Source: CAD feature listing. Evaluate the final solid. Frame: model axes, mm. A direction names the side the tool comes from. Coordinates: 2 decimals unless noted, no trailing zeros. Write each loop counter-clockwise with the first axis right and the second up, starting at its lowest first coordinate (ties: lowest second). Pieces come first, ordered by that corner, then holes. Notation, with made-up numbers: M 68,44.25 L 102,44.25 A24 cw 102,56.25 Z; hole C -28,79 d6. An arc over 180 degrees is marked long. Write item = value, one per line. Start each with the question number.
1. Section query A-A (z = 9.75). Output: boundary loops of the cut face in (x, y).
2. Pin query (flat end, axial travel): pin 1 Ø17.5 at (y, z) = (-6.5, 8.5) entering from +X; pin 2 Ø11 at (x, z) = (3.5, -5) entering from -Y; pin 3 Ø13 at (x, z) = (14, -4) entering from +Y; pin 4 Ø6 at (y, z) = (-43, 1) entering from -X. Return the tip coordinate at first contact, or that it passes through.
3. Section query D-D (z = -7.75). Output: boundary loops of the cut face in (x, y).
4. Pull-direction query (X, two-part tool) for faces 1 (the face through (59, -16.4, 1)), 2 (the face through (82.6, 20.5, 1.6)), 3 (the face through (48.612, 22.153, 1.158)); classes: pulls with the +X half, pulls with the -X half, needs draft (parallel to the pull), parting line crosses it, or undercut.
5. Line query: line 1 along X through (y, z) = (-21.5, 8.5); line 2 along Y through (x, z) = (35, -8); line 3 along Z through (x, y) = (57, 6). Output: solid intervals per line, ascending.
6. Section query B-B (x = 44). Output: boundary loops of the cut face in (y, z), then the cut area to 3 significant figures.
7. Section query C-C (y = -82.5). Output: boundary loops of the cut face in (x, z), then the cut area to 3 significant figures.
8. Access query for faces 4 (the face through (81.4, -20.5, 1.6)), 5 (the face through (88, 24, 10)), 6 (the face through (-59, -16.4, 1)). Directions: +Z, -Z, +X, -X, +Y, -Y. A direction counts if a zero-diameter tool reaches every point of the face in a straight line with its end or side. Return the directions, or none.
```python
from build123d import *

# Parameters (mm, degrees)
F0_W      = 56
F0_H      = 16
F1_DEPTH  = 27.5
F2_DEPTH  = 15
F4_DEPTH  = 30.001
F6_DEPTH  = 18
F9_D      = 2.5
F9_DEPTH  = 12
F9_TIP    = 0.7510757738
F11_DEPTH = 2


with BuildPart() as f1:
    # F0 (on Front) → F1 (new body, symmetric)
    with BuildSketch(Plane.XZ):
        Polygon((-30, 20), (-90, 20), (-90, 0), (-55, 0), (-30, 0), align=None)
        with Locations((-60, 10)):
            Rectangle(F0_W, F0_H, mode=Mode.SUBTRACT)
    extrude(amount=F1_DEPTH, both=True)


with BuildPart() as f1b:
    # F0 (on Front) → F1, piece 2 (new body, symmetric)
    with BuildSketch(Plane.XZ):
        Polygon((30, 20), (30, 0), (55, 0), (90, 0), (90, 20), align=None)
        with Locations((60, 10)):
            Rectangle(F0_W, F0_H, mode=Mode.SUBTRACT)
    extrude(amount=F1_DEPTH, both=True)


with BuildPart() as f2:
    # F0 (on Front) → F2 (new body, symmetric)
    with BuildSketch(Plane.XZ):
        Polygon((30, 0), (-30, 0), (-55, 0), (-55, -1), (-46, -10), (46, -10), (55, -1), (55, 0), align=None)
    extrude(amount=F2_DEPTH, both=True)

    # F10 (on face) → F11 (join)
    with BuildSketch(Plane.XY):
        Polygon((28.5, 15), (-28.5, 15), (-28.5, -27), (-19.5, -78), (-19.5, -115), (19.5, -115), (19.5, -78), (28.5, -27), align=None)
    extrude(amount=F11_DEPTH)


with BuildPart() as f4_tool:
    # F3 (on face) → F4 (new body, through all)
    with BuildSketch(Plane.XY.offset(20)):
        Polygon((-30, 27.5), (-70, 27.5), (-30, 17.5), align=None)
        Polygon((-70, -27.5), (-30, -27.5), (-30, -17.5), align=None)
        Polygon((30, 17.5), (70, 27.5), (30, 27.5), align=None)
        Polygon((70, -27.5), (30, -17.5), (30, -27.5), align=None)
    extrude(amount=-F4_DEPTH)


with BuildPart() as f1_1:
    add(f1.part)

    # F4: cut by f4_tool
    add(f4_tool.part, mode=Mode.SUBTRACT)

    # F5 (on face) → F6 (cut, through all)
    with BuildSketch(Plane(origin=(0, 0, 0), x_dir=(1, 0, 0), z_dir=(0, 0, -1))):
        with BuildLine():
            Line((-63, 20.5), (-90, 20.5))
            Line((-90, 20.5), (-90, -20.5))
            Line((-90, -20.5), (-63, -20.5))
            ThreePointArc((-63, -20.5), (-59, -16.5), (-63, -12.5))
            Line((-63, -12.5), (-63, 12.5))
            ThreePointArc((-63, 12.5), (-59, 16.5), (-63, 20.5))
        make_face()
    extrude(amount=-F6_DEPTH, mode=Mode.SUBTRACT)

    # F9
    with Locations(Plane(origin=(-90, 0, 0), x_dir=(0, -1, 0), z_dir=(-1, 0, 0))):
        with Locations((-24.2568291724, 14.9830980226), (-24.2568291724, 2.1462233271), (24.2568291724, 14.9830980226), (24.2568291724, 2.1462233271)):
            Hole(F9_D / 2, depth=F9_DEPTH)
            with Locations((0, 0, -(F9_DEPTH + F9_TIP / 2))):  # 118° drill point
                Cone(0, F9_D / 2, F9_TIP, mode=Mode.SUBTRACT)



with BuildPart() as f1b_1:
    add(f1b.part)

    # F4: cut by f4_tool
    add(f4_tool.part, mode=Mode.SUBTRACT)


with BuildPart() as f1_2:
    add(f1_1.part)

    add(f2.part)  # F12 merges F2
    # F12: F1 across plane
    add(f1_1.part.mirror(Plane.YZ))


solid = f1_2.part
```
Results are:
q1.outline = M -90,-27.5 L -88,-27.5 L -88,-20.5 L -90,-20.5 Z; M -90,20.5 L -88,20.5 L -88,27.5 L -90,27.5 Z; M -32,-18 L -30,-17.5 L -30,17.5 L -32,18 Z; M 30,-17.5 L 32,-18 L 32,18 L 30,17.5 Z; M 88,-27.5 L 90,-27.5 L 90,-20.5 L 88,-20.5 Z; M 88,20.5 L 90,20.5 L 90,27.5 L 88,27.5 Z
q2.pin_1 = 63
q2.pin_2 = -115
q2.pin_3 = 15
q2.pin_4 = -26.21
q3.outline = M -48.25,-15 L 48.25,-15 L 48.25,15 L -48.25,15 Z
q4.face_1 = pulls with the +X half
q4.face_2 = needs draft
q4.face_3 = undercut
q5.line_1 = -90 to -88, 88 to 90
q5.line_2 = -15 to 15
q5.line_3 = 0 to 2, 18 to 20
q6.outline = M -21,0 L -15,0 L -15,-10 L 15,-10 L 15,0 L 21,0 L 21,2 L -21,2 Z; M -21,18 L 21,18 L 21,20 L -21,20 Z
q6.area = 468 mm^2
q7.outline = M -19.5,0 L 19.5,0 L 19.5,2 L -19.5,2 Z
q7.area = 78.0 mm^2
q8.face_4 = -Z, +X
q8.face_5 = +Y, -Y
q8.face_6 = -Z, -X
